from build123d import *

# Parameters (mm, degrees)
F0_W     = 20
F0_H     = 25
F0_W_2   = 17.5
F0_H_2   = 22.5
F0_W_3   = 37.5
F0_W_4   = 35
F0_H_3   = 32.5
F0_W_5   = 22.5
F0_H_4   = 35
F1_DEPTH = 25
F2_W     = 60
F2_H     = 0.691662
F3_DEPTH = 39
F4_DEPTH = 21


with BuildPart() as f1:
    # F0 (on Top) → F1 (new body)
    with BuildSketch(Plane.XY):
        with Locations((-56.303288, 26.577459)):
            Rectangle(F0_W, F0_H)
        with Locations((-56.396089, 26.54361)):
            Rectangle(F0_W_2, F0_H_2, mode=Mode.SUBTRACT)
        Polygon((-6.303288, 39.077459), (-46.303288, 39.077459), (-46.303288, 14.077459), (-28.803288, 14.077459), (-6.303288, 14.077459), align=None)
        with Locations((-26.331019, 26.54361)):
            Rectangle(F0_W_3, F0_H_2, mode=Mode.SUBTRACT)
        Polygon((-28.803288, 14.077459), (-46.303288, 14.077459), (-66.303288, 14.077459), (-66.303288, -20.922541), (-28.803288, -20.922541), align=None)
        with Locations((-47.646089, -3.499608)):
            Rectangle(F0_W_4, F0_H_3, mode=Mode.SUBTRACT)
        with Locations((-17.553288, -3.422541)):
            Rectangle(F0_W_5, F0_H_4)
        with Locations((-17.418107, -3.217003)):
            Rectangle(F0_W, F0_H_3, mode=Mode.SUBTRACT)
    extrude(amount=F1_DEPTH)

    # F2 (on Front) → F3 (join)
    with BuildSketch(Plane.XZ):
        with Locations((-36.265093, -0.345831)):
            Rectangle(F2_W, F2_H)
    extrude(amount=-F3_DEPTH)

    # F3_face (on face) → F4 (join)
    with BuildSketch(Plane(origin=(-36.265093, 0, -0.345831), x_dir=(1, 0, 0), z_dir=(0, -1, 0))):
        Polygon((30, -0.345831), (30, 0.345831), (29.961805, 0.345831), (28.846987, 0.345831), (8.846987, 0.345831), (6.119005, 0.345831), (-28.880995, 0.345831), (-30, 0.345831), (-30, -0.345831), align=None)
    extrude(amount=F4_DEPTH)


solid = f1.part
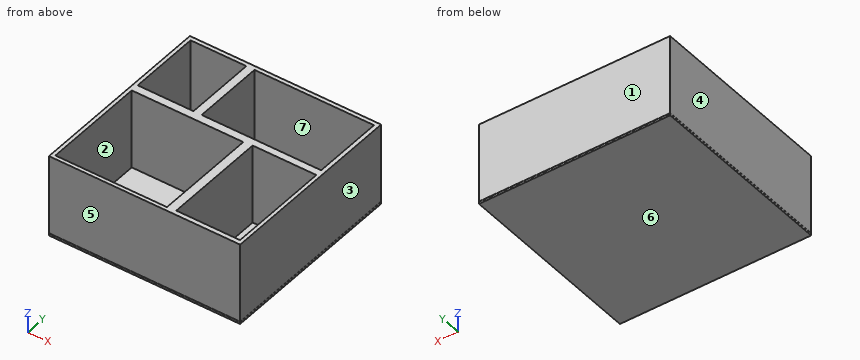
Could you check a few things on this model? Use its own coordinates, in mm. Face numbers are marked on the shaded views. A direction names the side the tool comes from. Coordinates: 2 decimals unless noted, no trailing zeros. Order: outer loops, then holes, each group sorted by start corner. A loop starts at its lowest first (then second) coordinate and runs counter-clockwise, first axis right, second up. Notation, with made-up numbers: (27.5, 50) -> (35.5, 50) arc R8 cw to (35.5, 61) -> close; hole circle Ø3 at (-33.75, 18.5). An arc over 180 degrees is marked (long way). One line per item, written item: value. Start each with the question number.
1) Imagine slicing it at A-A on z = 20.75. List the corners of the cut face in (x, y) for me, plus the area to 3 significant figures.
2) If I drill on L1, parallel to X at y = 22.5, z = 15.25; L2, parallel to Y at x = -24, z = 23; L3, parallel to X at y = -8, z = 20.5, over which ranges is the centre line in solid material (lowest first)? Write a range as [from, to].
3) Imagine slicing it at B-B on x = -46. List the corners of the cut face in (y, z) for me.
4) I'm going to push flat-ended pins straight in: pin 1 (6 mm diameter, centred on x = -15.5, y = 24.5, fed in from +Z); pin 2 (6 mm diameter, centred on x = -32, z = 20.5, fed in from -Y); pin 3 (8 mm diameter, centred on y = -6, z = 2.5, fed in from +X); pin 4 (0.6 mm diameter, centred on x = -45.5, z = -0.5, fed in from +Y). Where does each tip first touch, or does it pass through?
5) Imagine slicing it at D-D on x = -17. List the corners of the cut face in (y, z) for me.
6) Which directions (+Z, -Z, +X, -X, +Y, -Y) give clear straight access to the entire face, cutting with the end or side of a thin tool? Please do the marked faces 5, 6 and 7.
7) We'd pull the mould along X, two halves only. Please class the marked faces 1, 2, 3 and 4: +X half, -X half, draft (parallel to the pull), parting line (faces both ways), or undercut.
Answer list:
1. outline: (-66.3, -20.92) -> (-6.3, -20.92) -> (-6.3, 39.08) -> (-66.3, 39.08) -> close; hole (-65.15, -19.75) -> (-30.15, -19.75) -> (-30.15, 12.75) -> (-65.15, 12.75) -> close; hole (-65.15, 15.29) -> (-47.65, 15.29) -> (-47.65, 37.79) -> (-65.15, 37.79) -> close; hole (-45.08, 15.29) -> (-7.58, 15.29) -> (-7.58, 37.79) -> (-45.08, 37.79) -> close; hole (-27.42, -19.47) -> (-7.42, -19.47) -> (-7.42, 13.03) -> (-27.42, 13.03) -> close
1. area: 575 mm2
2. L1: x = [-66.3, -65.15], [-47.65, -45.08], [-7.58, -6.3]
2. L2: y = [-20.92, -19.47], [13.03, 15.29], [37.79, 39.08]
2. L3: x = [-66.3, -65.15], [-30.15, -27.42], [-7.42, -6.3]
3. outline: (-21, -0.69) -> (39, -0.69) -> (39, 0) -> (39.08, 0) -> (39.08, 25) -> (12.75, 25) -> (12.75, 0) -> (-19.75, 0) -> (-19.75, 25) -> (-20.92, 25) -> (-20.92, 0) -> (-21, 0) -> close
4. pin 1: stops at z = 0
4. pin 2: stops at y = -20.92
4. pin 3: stops at x = -6.27
4. pin 4: stops at y = 39
5. outline: (-21, -0.69) -> (39, -0.69) -> (39, 0) -> (39.08, 0) -> (39.08, 25) -> (37.79, 25) -> (37.79, 0) -> (15.29, 0) -> (15.29, 25) -> (13.03, 25) -> (13.03, 0) -> (-19.47, 0) -> (-19.47, 25) -> (-20.92, 25) -> (-20.92, 0) -> (-21, 0) -> close
6. face 5: +Z, +X, -X, -Y
6. face 6: -Z, +X, -X, +Y, -Y
6. face 7: +Z
7. face 1: draft
7. face 2: undercut
7. face 3: +X half
7. face 4: -X half
